Input: part model. Units: mm. Frame: model coordinates. A direction names the side the tool comes from. Give positions to 0.01 mm unless a question says otherwise; leave off trailing zeros. Order: outer loops, then holes, each group sorted by start corner. A loop starts at its lowest first (then second) coordinate and runs counter-clockwise, first axis right, second up.
```python
from build123d import *

# Parameters (mm, degrees)
TABAN_FLAN_1_DEPTH = 1110
SEKME1_DEPTH       = 8


# Sheet-metal steps are written as plain solids
with BuildPart() as part:
    # Çizim1 → Taban-Flanş1 (new body)
    with BuildSketch(Plane.XY):
        with BuildLine():
            Line((0, 0), (5.960525983, -55.31134025))
            ThreePointArc((5.960525983, -55.31134025), (11.177974486, -65.501435482), (21.868424162, -69.597054535))
            Line((21.868424162, -69.597054535), (271.131575838, -69.597054535))
            ThreePointArc((271.131575838, -69.597054535), (281.822025514, -65.501435482), (287.039474017, -55.31134025))
            Line((287.039474017, -55.31134025), (293, 0))
            Line((293, 0), (285.04605091, 0.857142857))
            Line((285.04605091, 0.857142857), (279.085524928, -54.454197393))
            ThreePointArc((279.085524928, -54.454197393), (276.476800676, -59.549245009), (271.131575838, -61.597054535))
            Line((271.131575838, -61.597054535), (21.868424162, -61.597054535))
            ThreePointArc((21.868424162, -61.597054535), (16.523199324, -59.549245009), (13.914475072, -54.454197393))
            Line((13.914475072, -54.454197393), (7.95394909, 0.857142857))
            Line((7.95394909, 0.857142857), (0, 0))
        make_face()
    extrude(amount=TABAN_FLAN_1_DEPTH)

    # Çizim6 → Sekme1 (add)
    with BuildSketch(Plane(origin=(0, -61.597054535, 0), x_dir=(1, 0, 0), z_dir=(0, 1, 0))):
        Polygon((62, 0), (146.5, 135.866662578), (231, 0), align=None)
    extrude(amount=-SEKME1_DEPTH)


solid = part.part
```
1) Cut plane C-C (x = 260.5). Return the cut outline in (y, z).
2) Reachability of faces 4 (the face through (146, -63, 1110)), 5 (the face through (280, -50, 0)), 6 (the face through (10.976, -27.186, 547.23)) from +Z, -Z, +X, -X, +Y, -Y: full face, straight path, thin tool, end or side. Return the list, or none.
3) Line query: probe 1 along Y at (x, z) = (196, 196.5); probe 2 along X at (y, z) = (-4, 151.5); probe 3 along X at (y, z) = (-23, 601.5). Output: solid intervals per line, ascending.
4) Cut plane B-B (y = -35.5). Return the cut outline in (x, z), then the cut area to 3 significant figures.
5) First-contact query: P1, Ø18.5, axis at x = 264, y = -25, coming from the -Z side; P2, Ø1, axis at y = -39.5, z = 62, coming from the +X side; P3, Ø1, axis at x = 214.5, z = 303.5, coming from the +Y side; P4, Ø4, axis at y = -11.5, z = 87.5, coming from the -X side. Flat tips, straight axial feed; report the tip coordinate or a pass-through.
6) Pull-direction query (X, two-part tool) for faces 1 (the face through (148, -61.597, 478)), 2 (the face through (289.98, -28.04, 547.23)), 3 (the face through (12, -47, 0)); classes: pulls with the +X half, pulls with the -X half, needs draft (parallel to the pull), parting line crosses it, or undercut.
7) Cut plane D-D (z = -25). Return the cut outline in (x, y).
8) Cut plane A-A (z = 895). Return the cut outline in (x, y), then the cut area to 3 significant figures.
Geometry says:
1. outline: (-69.6, 0) - (-61.6, 0) - (-61.6, 1110) - (-69.6, 1110) - close
2. face 4: +Z, +X, -X, +Y, -Y
2. face 5: -Z, +X, +Y, -Y
2. face 6: +Z, -Z, +Y
3. probe 1: y = -69.6 to -61.6
3. probe 2: x = 0.43 to 8.48, 284.52 to 292.57
3. probe 3: x = 2.48 to 10.52, 282.48 to 290.52
4. outline: (3.83, 0) - (11.87, 0) - (11.87, 1110) - (3.83, 1110) - close; (281.13, 0) - (289.17, 0) - (289.17, 1110) - (281.13, 1110) - close
4. area: 17,900 mm2
5. P1: passes through
5. P2: stops at x = 288.8
5. P3: stops at y = -61.6
5. P4: stops at x = 1.02
6. face 1: undercut
6. face 2: pulls with the +X half
6. face 3: needs draft
7. outline: (77.55, -69.6) - (215.45, -69.6) - (215.45, -61.6) - (77.55, -61.6) - close
8. outline: (0, 0) - (5.96, -55.31) arc R16 ccw to (21.87, -69.6) - (271.13, -69.6) arc R16 ccw to (287.04, -55.31) - (293, 0) - (285.05, 0.86) - (279.09, -54.45) arc R8 cw to (271.13, -61.6) - (21.87, -61.6) arc R8 cw to (13.91, -54.45) - (7.95, 0.86) - close
8. area: 3,170 mm2
